Read the model definition and answer for the solid it produces. Units are mm, in the model's axes. Round coordinates to 2 decimals unless told otherwise and drop trailing zeros. Write each loop counter-clockwise with the first axis right and the second up, starting at its lowest first coordinate (ties: lowest second). Pieces come first, ordered by that corner, then holes.
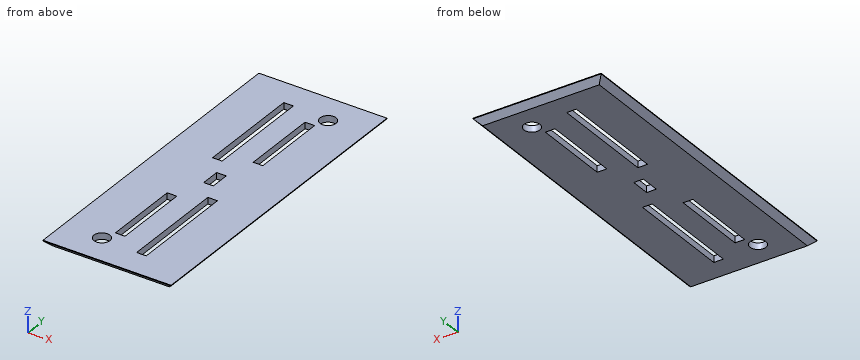
from build123d import *

# Parameters (mm, degrees)
SKETCH_W     = 40
SKETCH_H     = 100
SKETCH_R     = 2.5
SKETCH_W_2   = 3
SKETCH_H_2   = 33
SKETCH_H_3   = 24
SKETCH_H_4   = 6
PAD_DEPTH    = 2
CHAMFER_SIZE = 1.8


with BuildPart() as part:
    # Sketch → Pad (new body)
    with BuildSketch(Plane.XY):
        Rectangle(SKETCH_W, SKETCH_H)
        with Locations((-8, -40.5)):
            Circle(SKETCH_R, mode=Mode.SUBTRACT)
        with Locations((8, 40.5)):
            Circle(SKETCH_R, mode=Mode.SUBTRACT)
        with Locations((-5, 25)):
            Rectangle(SKETCH_W_2, SKETCH_H_2, mode=Mode.SUBTRACT)
        with Locations((5, -25)):
            Rectangle(SKETCH_W_2, SKETCH_H_2, mode=Mode.SUBTRACT)
        with Locations((5, 24.5)):
            Rectangle(SKETCH_W_2, SKETCH_H_3, mode=Mode.SUBTRACT)
        with Locations((-5, -24.5)):
            Rectangle(SKETCH_W_2, SKETCH_H_3, mode=Mode.SUBTRACT)
        Rectangle(SKETCH_W_2, SKETCH_H_4, mode=Mode.SUBTRACT)
    extrude(amount=PAD_DEPTH)

    # Chamfer
    chamfer_edges = [part.edges().sort_by_distance(p)[0] for p in [
        (0, -50, 0),
        (20, 0, 0),
        (0, 50, 0),
        (-20, 0, 0),
    ]]
    chamfer(chamfer_edges, length=CHAMFER_SIZE)


solid = part.part
Q1. Section A-A (z = 1.45) is taken. Determine the outline of the cut face in (x, y), then the cut area to 3 significant figures.
Verdict:
outline: (-19.65, -49.65) - (19.65, -49.65) - (19.65, 49.65) - (-19.65, 49.65) - close; hole circle Ø5 at (-8, -40.5); hole (-6.5, -36.5) - (-3.5, -36.5) - (-3.5, -12.5) - (-6.5, -12.5) - close; hole (-6.5, 8.5) - (-3.5, 8.5) - (-3.5, 41.5) - (-6.5, 41.5) - close; hole (-1.5, -3) - (1.5, -3) - (1.5, 3) - (-1.5, 3) - close; hole (3.5, -41.5) - (6.5, -41.5) - (6.5, -8.5) - (3.5, -8.5) - close; hole (3.5, 12.5) - (6.5, 12.5) - (6.5, 36.5) - (3.5, 36.5) - close; hole circle Ø5 at (8, 40.5)
area: 3,500 mm2
Q2. Section C-C (x = -8) is taken. Determine the outline of the cut face in (y, z).
Verdict:
outline: (-50, 1.8) - (-48.2, 0) - (-43, 0) - (-43, 2) - (-50, 2) - close; (-38, 0) - (48.2, 0) - (50, 1.8) - (50, 2) - (-38, 2) - close
Q3. Flat-ended cylindrical pins translate along their axes: pin 1 Ø1 at (x, z) = (5.5, 1) entering from -Y; pin 2 Ø0.6 at (x, z) = (4.5, 1) entering from -Y; pin 3 Ø0.6 at (y, z) = (17.5, 1) entering from -X. Find the tip coordinate at first contact, or state that the pin passes through.
Verdict:
pin 1: stops at y = -49.7
pin 2: stops at y = -49.5
pin 3: stops at x = -19.5
Q4. Section D-D (y = -29.5) is taken. Determine the outline of the cut face in (x, z).
Verdict:
outline: (-20, 1.8) - (-18.2, 0) - (-6.5, 0) - (-6.5, 2) - (-20, 2) - close; (-3.5, 0) - (3.5, 0) - (3.5, 2) - (-3.5, 2) - close; (6.5, 0) - (18.2, 0) - (20, 1.8) - (20, 2) - (6.5, 2) - close
Q5. Straight lines are drawn through the part: probe 1 along X at (y, z) = (17.5, 1.9); probe 2 along X at (y, z) = (-41, 0.85); probe 3 along Y at (x, z) = (-9, 1.5). For each, find the intervals that lie inside material, in ascending order.
Verdict:
probe 1: x = -20 to -6.5, -3.5 to 3.5, 6.5 to 20
probe 2: x = -19.05 to -10.45, -5.55 to 3.5, 6.5 to 19.05
probe 3: y = -49.7 to -42.79, -38.21 to 49.7
Q6. Section B-B (y = -9.5) is taken. Determine the outline of the cut face in (x, z).
Verdict:
outline: (-20, 1.8) - (-18.2, 0) - (3.5, 0) - (3.5, 2) - (-20, 2) - close; (6.5, 0) - (18.2, 0) - (20, 1.8) - (20, 2) - (6.5, 2) - close
